Could you check a few things on this model? Use its own coordinates, in mm. A direction names the side the tool comes from. Give positions to 0.01 mm unless a question says otherwise; leave off trailing zeros. Order: outer loops, then holes, each group sorted by start corner. A loop starts at its lowest first (then second) coordinate and runs counter-clockwise, first axis right, second up. Notation, with made-up numbers: M 41.5,6 L 99.5,6 A18 ccw 99.5,32 Z; hole C 38,-32 d5. An arc over 180 degrees is marked long. Use a Markdown table: item, result. Add a question column.
Item 1: For faces 4 (the face through (-22.9, 22.714, 3.131)), 5 (the face through (-23.03, -6.72, 3.13)), 6 (the face through (8, 6.156, 3)), 7 (the face through (-30, 6.156, 3)), which set-ups out of +Z, -Z, +X, -X, +Y, -Y let a thin tool reach every point of the face, with its end or its side?
Item 2: If I drill on L1, parallel to X at y = 25.5, z = 2.75; L2, parallel to Y at x = 5, z = 1.5; L3, parallel to X at y = -2.5, z = 5, over which ranges is the centre line in solid material (lowest first)? Write a range as from..to.
Item 3: Suppose I cut it at B-B on y = 19.5. Write out the boundary of the cut face in (x, z).
Item 4: Suppose I cut it at A-A on x = -8. Write out the boundary of the cut face in (y, z).
Item 5: Suppose I cut it at D-D on x = 2.5. Write out the boundary of the cut face in (y, z), plus the area to 3 significant figures.
Item 6: I'm going to push flat-ended pins straight in: pin 1 Ø3 at (y, z) = (20.5, 5.5) entering from +X; pin 2 Ø1 at (y, z) = (21, 1.5) entering from -X; pin 3 Ø3 at (y, z) = (29.5, 2.5) entering from -X. Where does each tip first touch, or does it pass through?
Item 7: If we mould it in two halves opening along X, with no side actions, what happens to faces 1 (the face through (-36.198, 8, 3)), 2 (the face through (14.315, 8, 3)), 3 (the face through (-9.036, -11, 3))? For each: released by +X, released by -X, zero draft, split by the parting line, or undercut.
from build123d import *

# Parameters (mm, degrees)
F0_R     = 9.525
F1_DEPTH = 6.35
F2_COUNT = 8


with BuildPart() as f1:
    # F0 (on Top) → F1 (new body)
    with BuildSketch(Plane.XY):
        with BuildLine():
            ThreePointArc((-12.8463400356, 20.6174660121), (-19.2207270902, -1.5690979595), (1.7586599644, 8.0611538545))
            ThreePointArc((1.7586599644, 8.0611538545), (-1.3110882217, 16.3405409091), (-9.0363400356, 20.6174660121))
            Line((-9.0363400356, 20.6174660121), (-12.8463400356, 20.6174660121))
        make_face()
        with Locations((-10.9413400356, 8.0611538545)):
            Circle(F0_R, mode=Mode.SUBTRACT)
        with BuildLine():
            Line((-12.8463400356, 20.6174660121), (-9.0363400356, 20.6174660121))
            ThreePointArc((-9.0363400356, 20.6174660121), (-10.9413400356, 20.7611538545), (-12.8463400356, 20.6174660121))
        make_face()
        with BuildLine():
            ThreePointArc((-12.8463400356, 20.6174660121), (-10.9413400356, 20.7611538545), (-9.0363400356, 20.6174660121))
            Line((-9.0363400356, 20.6174660121), (-9.0363400356, 33.3174660121))
            Line((-9.0363400356, 33.3174660121), (-12.8463400356, 33.3174660121))
            Line((-12.8463400356, 33.3174660121), (-12.8463400356, 20.6174660121))
        make_face()
    extrude(amount=F1_DEPTH)

    # F2: F1 ×8 about axis
    f2_axis = Axis((-10.9413400356, 8.0611538545, 6.35), (0, 0, 1))


with BuildPart() as f1_1:
    add(f1.part)
    for i in range(1, F2_COUNT):
        add(f1.part.rotate(f2_axis, i * 360 / F2_COUNT))


solid = f1_1.part
Findings below:
| question | item | result |
|---|---|---|
| 1 | face 4 | +Z, -Z, +Y |
| 1 | face 5 | +Z, -Z, -Y |
| 1 | face 6 | +Z, -Z, +X |
| 1 | face 7 | +Z, -Z, -X |
| 2 | L1 | x = -29.22..-25.69, -12.85..-9.04, 3.8..7.34 |
| 2 | L2 | y = -10.57..-5.19, 6.16..9.97, 21.31..26.7 |
| 2 | L3 | x = -24.2..-18.81, -17.99..-3.89, -3.07..2.31 |
| 3 | outline | M -25.07,0 L -19.69,0 L -19.69,6.35 L -25.07,6.35 Z; M -16.46,0 L -5.42,0 L -5.42,6.35 L -16.46,6.35 Z; M -2.2,0 L 3.19,0 L 3.19,6.35 L -2.2,6.35 Z |
| 4 | outline | M -4.29,0 L -1,0 L -1,6.35 L -4.29,6.35 Z; M 17.12,0 L 20.42,0 L 20.42,6.35 L 17.12,6.35 Z |
| 5 | outline | M -8.07,0 L -2.69,0 L -2.69,6.35 L -8.07,6.35 Z; M 6.16,0 L 9.97,0 L 9.97,6.35 L 6.16,6.35 Z; M 18.81,0 L 24.2,0 L 24.2,6.35 L 18.81,6.35 Z |
| 5 | area | 92.6 mm^2 |
| 6 | pin 1 | stops at x = 5.69 |
| 6 | pin 2 | stops at x = -27.07 |
| 6 | pin 3 | stops at x = -12.85 |
| 7 | face 1 | released by -X |
| 7 | face 2 | released by +X |
| 7 | face 3 | undercut |
